Geometry: see drawing. Coordinates: mm, zero at the bounding-box minimum. Round coordinates to 2 decimals unless told otherwise and drop trailing zeros. Loops run counter-clockwise (first coordinate to the right, second up) from the corner with the lowest first, then second, coordinate; pieces in that order, holes last. Notation, with made-up numbers: (-24.5, 63.5) -> (-18.5, 63.5) arc R14 cw to (-18.5, 80.5) -> close; hole circle Ø1 at (-16.5, -31.75). An arc over 180 degrees is marked (long way). Answer in a Markdown table with one row per item.
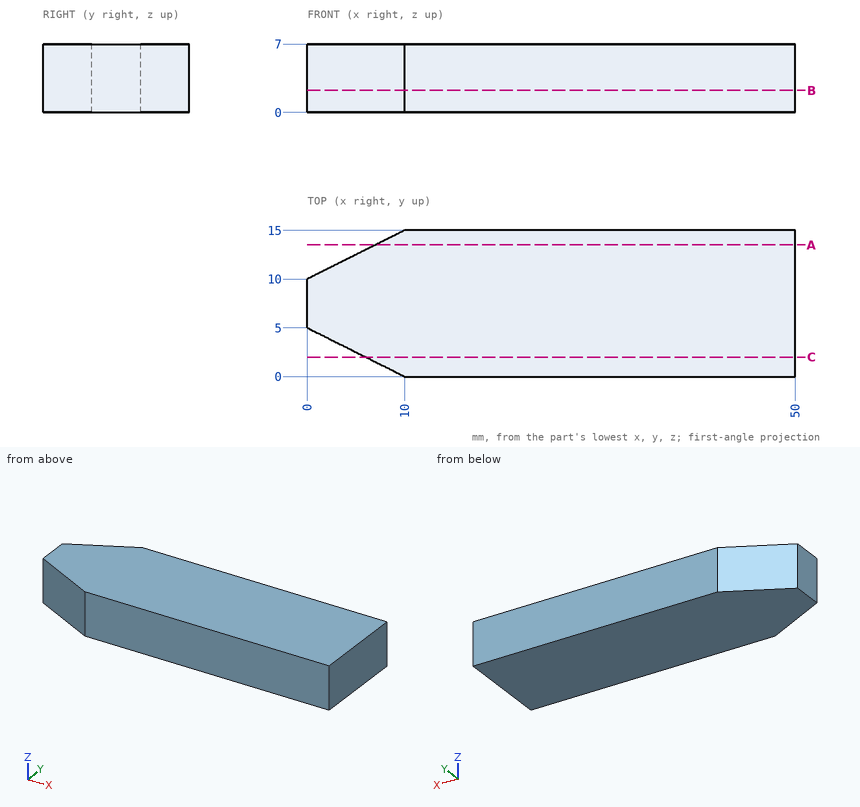
Item 1: Section query A-A, the plane y = 13.5. Output: boundary loops of the cut face in (x, z), and give its area (3 significant figures).
Ans:
| item | result |
|---|---|
| outline | (7, 0) -> (50, 0) -> (50, 7) -> (7, 7) -> close |
| area | 301 mm2 |
Item 2: Ray query, L1, parallel to X at y = 4.5, z = 5.5; L2, parallel to X at y = 3.5, z = 1.75; L3, parallel to Y at x = 2, z = 5.75. Return the intervals inside material, ascending.
Ans:
| item | result |
|---|---|
| L1 | 1 to 50 |
| L2 | 3 to 50 |
| L3 | 4 to 11 |
Item 3: Section query B-B, the plane z = 2.25. Output: boundary loops of the cut face in (x, y).
Ans:
| item | result |
|---|---|
| outline | (0, 5) -> (10, 0) -> (50, 0) -> (50, 15) -> (10, 15) -> (0, 10) -> close |
Item 4: Section query C-C, the plane y = 2. Output: boundary loops of the cut face in (x, z), and give its area (3 significant figures).
Ans:
| item | result |
|---|---|
| outline | (6, 0) -> (50, 0) -> (50, 7) -> (6, 7) -> close |
| area | 308 mm2 |
